from build123d import *

# Parameters (mm, degrees)
SKETCH1_W       = 36
SKETCH1_H       = 40
EXTRUDE1_DEPTH  = 5
EXTRUDE2_DEPTH  = 5
EXTRUDE3_DEPTH  = 5
SKETCH4_R       = 3
EXTRUDE4_DEPTH  = 3
SKETCH5_R       = 1.6
EXTRUDE5_DEPTH  = 3
EXTRUDE6_START  = 6
SKETCH6_R       = 3
EXTRUDE6_DEPTH  = 6
FILLET1_R       = 2
EXTRUDE7_DEPTH  = 1
SKETCH9_R       = 1.6
EXTRUDE8_DEPTH  = 49.836461788
SKETCH10_R      = 3
EXTRUDE9_DEPTH  = 2
SKETCH11_R      = 3
EXTRUDE10_DEPTH = 39.118237105
FILLET2_R       = 2


with BuildPart() as part:
    # Sketch1 → Extrude1 (new body)
    with BuildSketch(Plane(origin=(0, 0, 0), x_dir=(1, 0, 0), z_dir=(0, 1, 0))):
        Rectangle(SKETCH1_W, SKETCH1_H)
    extrude(amount=EXTRUDE1_DEPTH)

    # Sketch2 → Extrude2 (add)
    with BuildSketch(Plane.ZY.offset(18)):
        Polygon((-20, 0), (-20, 32), (-12, 32), (20, 5), (20, 0), align=None)
    extrude(amount=-EXTRUDE2_DEPTH)

    # Sketch3 → Extrude3 (add)
    with BuildSketch(Plane(origin=(18, 0, 0), x_dir=(0, 0, -1), z_dir=(1, 0, 0))):
        Polygon((20, 0), (20, 32), (12, 32), (-20, 5), (-20, 0), align=None)
    extrude(amount=-EXTRUDE3_DEPTH)

    # Sketch4 → Extrude4 (cut)
    with BuildSketch(Plane(origin=(0, 5, 0), x_dir=(1, 0, 0), z_dir=(0, 1, 0))):
        with Locations(Location((-12, 12, 0), (0, 0, 270))):
            Circle(SKETCH4_R)
        with Locations(Location((-12, -12, 0), (0, 0, 270))):
            Circle(SKETCH4_R)
        with Locations(Location((12, 12, 0), (0, 0, 270))):
            Circle(SKETCH4_R)
        with Locations(Location((12, -12, 0), (0, 0, 270))):
            Circle(SKETCH4_R)
    extrude(amount=-EXTRUDE4_DEPTH, mode=Mode.SUBTRACT)

    # Sketch5 → Extrude5 (cut)
    with BuildSketch(Plane(origin=(0, 2, 0), x_dir=(1, 0, 0), z_dir=(0, 1, 0))):
        with Locations(Location((-12, 12, 0), (0, 0, 270))):
            Circle(SKETCH5_R)
        with Locations(Location((-12, -12, 0), (0, 0, 270))):
            Circle(SKETCH5_R)
        with Locations(Location((12, -12, 0), (0, 0, 270))):
            Circle(SKETCH5_R)
        with Locations(Location((12, 12, 0), (0, 0, 270))):
            Circle(SKETCH5_R)
    extrude(amount=-EXTRUDE5_DEPTH, mode=Mode.SUBTRACT)

    # Sketch6 → Extrude6 (cut)
    with BuildSketch(Plane(origin=(0, 5, 0), x_dir=(1, 0, 0), z_dir=(0, 1, 0)).offset(EXTRUDE6_START)):
        with Locations(Location((-12, 12, 0), (0, 0, 270))):
            Circle(SKETCH6_R)
        with Locations(Location((12, 12, 0), (0, 0, 270))):
            Circle(SKETCH6_R)
    extrude(amount=-EXTRUDE6_DEPTH, mode=Mode.SUBTRACT)

    # Fillet1
    fillet1_edges = [part.edges().sort_by_distance(p)[0] for p in [
        (-15.5, 32, -20),
        (-15.5, 32, -12),
        (15.5, 32, -20),
        (15.5, 32, -12),
    ]]
    fillet(fillet1_edges, radius=FILLET1_R)

    # Sketch7 → Extrude7 (add)
    with BuildSketch(Plane(origin=(-13, 0, 0), x_dir=(0, 0, -1), z_dir=(1, 0, 0))):
        Polygon((16, 29.600452322), (13.312994231, 26.913446553), (16, 24.226440785), (18.687005769, 26.913446553), align=None)
    extrude7 = extrude(amount=EXTRUDE7_DEPTH)

    # Sketch9 → Extrude8 (cut, through all)
    with BuildSketch(Plane(origin=(-13, 0, 0), x_dir=(0, 0, -1), z_dir=(1, 0, 0))):
        with Locations((12, 14.913446553)):
            Circle(SKETCH9_R)
    extrude8 = extrude(amount=-EXTRUDE8_DEPTH, mode=Mode.SUBTRACT)

    # Sketch10 → Extrude9 (cut)
    with BuildSketch(Plane.ZY.offset(18)):
        with Locations((-12, 14.913446553)):
            Circle(SKETCH10_R)
    extrude9 = extrude(amount=-EXTRUDE9_DEPTH, mode=Mode.SUBTRACT)

    # Mirror2: Extrude7, Extrude8, Extrude9 across plane
    add(extrude7.mirror(Plane(origin=(0, 0, 0), x_dir=(0, 0, 1), z_dir=(1, 0, 0))))
    add(extrude8.mirror(Plane(origin=(0, 0, 0), x_dir=(0, 0, 1), z_dir=(1, 0, 0))), mode=Mode.SUBTRACT)
    add(extrude9.mirror(Plane(origin=(0, 0, 0), x_dir=(0, 0, 1), z_dir=(1, 0, 0))), mode=Mode.SUBTRACT)

    # Sketch11 → Extrude10 (cut, through all)
    with BuildSketch(Plane(origin=(0, 5, 0), x_dir=(1, 0, 0), z_dir=(0, 1, 0))):
        with Locations(Location((-12, -12, 0), (0, 0, 270))):
            Circle(SKETCH11_R)
        with Locations(Location((12, -12, 0), (0, 0, 270))):
            Circle(SKETCH11_R)
    extrude(amount=EXTRUDE10_DEPTH, mode=Mode.SUBTRACT)

    # Fillet2
    fillet2_edges = [part.edges().sort_by_distance(p)[0] for p in [
        (-18, 32, -15.365512697),
        (-18, 15, -20),
        (-18, 31.414213562, -19.414213562),
        (-18, 31.87845228, -12.044427235),
        (18, 32, -15.365512697),
        (18, 15, -20),
        (18, 18.264291484, 4.279358242),
        (18, 31.414213562, -19.414213562),
        (18, 31.87845228, -12.044427235),
        (-18, 18.264291484, 4.279358242),
        (18, 2.5, 20),
        (-18, 2.5, 20),
    ]]
    fillet(fillet2_edges, radius=FILLET2_R)


solid = part.part
Part model, mm, in its own coordinate system. A direction names the side the tool comes from. Coordinates: 2 decimals unless noted, no trailing zeros. Order: outer loops, then holes, each group sorted by start corner. A loop starts at its lowest first (then second) coordinate and runs counter-clockwise, first axis right, second up.
(1) Tool access for faces 1 (the face through (-13.3, 2, -10.7)), 2 (the face through (12.07, 1.01, -13.6)), 3 (the face through (-13, 6, 16)): list every direction of +Z, -Z, +X, -X, +Y, -Y with a clear straight run to the whole face (end or side of a thin tool).
Check sheet entries:
face 1: none
face 2: -Y
face 3: +Z, -Z, +Y
(2) Probe L1, parallel to Z at x = -12, y = 4; L2, parallel to X at y = 1, z = -12; L3, parallel to X at y = 10, z = 4.5. List the from-to ranges inside material, lowest first.
Check sheet entries:
L1: z = -20 to -15, -9 to 9, 15 to 20
L2: x = -18 to -13.6, -10.4 to 10.4, 13.6 to 18
L3: x = -18 to -13, 13 to 18
(3) Pull direction X, two halves, no side cores. Call faces 4 (the face through (-15, 32, -15)), 5 (the face through (16, 13.6, -10.7)), 6 (the face through (-11.93, 1.01, 10.4)): pulls with the +X half, pulls with the -X half, needs draft (parallel to the pull), parting line crosses it, or undercut.
Check sheet entries:
face 4: needs draft
face 5: pulls with the +X half
face 6: undercut
(4) Slice it at B-B, the plane x = 3.5. Write the cut outline in (y, z), and give its area (3 significant figures).
Check sheet entries:
outline: (0, -20) - (5, -20) - (5, 20) - (0, 20) - close
area: 200 mm2
(5) Slice it at A-A, the plane z = -12. State how many separate pieces and enclosed holes the cut face has, and give its area (3 significant figures).
Check sheet entries:
separate pieces: 5
enclosed holes: 0
area: 331 mm2
(6) Pin check, flat tips, straight feed: pin 1 Ø4 at (y, z) = (14.91, -12) entering from +X; pin 2 Ø3 at (x, z) = (12.5, 11) entering from +Y. Stop position of each tip, or through.
Check sheet entries:
pin 1: stops at x = 16
pin 2: stops at y = 2
